The listing builds one solid part. Answer for the finished solid, in the listing's coordinates (mm). Face numbers are marked on the shaded views. A direction names the side the tool comes from. Coordinates: 2 decimals unless noted, no trailing zeros. Write each loop counter-clockwise with the first axis right and the second up, starting at its lowest first coordinate (ties: lowest second). Pieces come first, ordered by that corner, then holes. Notation, with made-up numbers: M 11,43 L 43,43 A37 cw 43,79 Z; hole C 70,77 d10. An arc over 180 degrees is marked long. Answer as CSV lines item,"result".
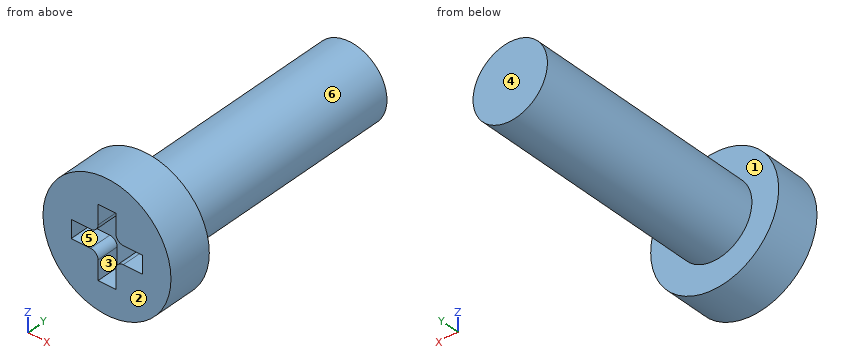
```python
from build123d import *

# Parameters (mm, degrees)
SKETCH_1_R          = 4.3
EXTRUDE_1_DEPTH     = 3
SKETCH_2_R          = 2.5
EXTRUDE_2_DEPTH     = 16
CUT_EXTRUDE_1_DEPTH = 1.5


with BuildPart() as part:
    # 草图1 → 凸台-拉伸1 (new body)
    with BuildSketch(Plane(origin=(0, 0, 0), x_dir=(1, 0, 0), z_dir=(0, 1, 0))):
        Circle(SKETCH_1_R)
    extrude(amount=EXTRUDE_1_DEPTH)

    # 草图2 → 凸台-拉伸2 (add)
    with BuildSketch(Plane(origin=(0, 3, 0), x_dir=(1, 0, 0), z_dir=(0, 1, 0))):
        Circle(SKETCH_2_R)
    extrude(amount=EXTRUDE_2_DEPTH)

    # 草图3 → 切除-拉伸1 (cut)
    with BuildSketch(Plane.XZ):
        with BuildLine():
            Line((-0.6, 1.1), (-0.6, 2.4))
            Line((-0.6, 2.4), (0.6, 2.4))
            Line((0.6, 2.4), (0.6, 1.1))
            ThreePointArc((0.6, 1.1), (0.746446609, 0.746446609), (1.1, 0.6))
            Line((1.1, 0.6), (2.4, 0.6))
            Line((2.4, 0.6), (2.4, -0.6))
            Line((2.4, -0.6), (1.1, -0.6))
            ThreePointArc((1.1, -0.6), (0.746446609, -0.746446609), (0.6, -1.1))
            Line((0.6, -1.1), (0.6, -2.4))
            Line((0.6, -2.4), (-0.6, -2.4))
            Line((-0.6, -2.4), (-0.6, -1.1))
            ThreePointArc((-0.6, -1.1), (-0.746446609, -0.746446609), (-1.1, -0.6))
            Line((-1.1, -0.6), (-2.4, -0.6))
            Line((-2.4, -0.6), (-2.4, 0.6))
            Line((-2.4, 0.6), (-1.1, 0.6))
            ThreePointArc((-1.1, 0.6), (-0.746446609, 0.746446609), (-0.6, 1.1))
        make_face()
    extrude(amount=-CUT_EXTRUDE_1_DEPTH, mode=Mode.SUBTRACT)


solid = part.part
```
Q1. Flat-ended cylindrical pins translate along their axes: pin 1 Ø5 at (x, y) = (1, 10.5) entering from -Z; pin 2 Ø1.5 at (x, y) = (-1, 7.5) entering from +Z; pin 3 Ø4 at (y, z) = (14, 3) entering from +X. Find the tip coordinate at first contact, or state that the pin passes through.
Output:
pin 1,"z = -2.5"
pin 2,"z = 2.49"
pin 3,"x = 2.29"
Q2. The mould has two halves that part along Z. Classify the marked faces 3, 4, 5 and 6: pulls with the +Z half, pulls with the -Z half, needs draft (parallel to the pull), parting line crosses it, or undercut.
Output:
face 3,"undercut"
face 4,"needs draft"
face 5,"undercut"
face 6,"parting line crosses it"
Q3. Find section D-D (z = 3.25). Give the vertices of the cut face in (x, y), and give its area (3 significant figures).
Output:
outline,"M -2.82,0 L 2.82,0 L 2.82,3 L -2.82,3 Z"
area,"16.9 mm2"
Q4. Straight lines are drawn through the part: line 1 (Y direction, x = -3, z = 3); line 2 (Y direction, x = -0.5, z = 0); line 3 (Z direction, x = 0, y = 8). For each, find the intervals that lie inside material, in ascending order.
Output:
line 1,"0 to 3"
line 2,"1.5 to 19"
line 3,"-2.5 to 2.5"
Q5. Find section C-C (y = 14.75). Give the vertices of the cut face in (x, z), and give its area (3 significant figures).
Output:
outline,"C 0,0 d5"
area,"19.6 mm2"
Q6. Find section B-B (z = 0). Give the vertices of the cut face in (x, y).
Output:
outline,"M -4.3,0 L -2.4,0 L -2.4,1.5 L 2.4,1.5 L 2.4,0 L 4.3,0 L 4.3,3 L 2.5,3 L 2.5,19 L -2.5,19 L -2.5,3 L -4.3,3 Z"
Q7. For the marked faces 1 and 2, determine the directions among +Z, -Z, +X, -X, +Y, -Y from which every point of the face is accessible in a straight line to the end or side of a thin tool.
Output:
face 1,"+Y"
face 2,"+Z, -Z, +X, -X, -Y"
Q8. Find section A-A (x = 0). Give the vertices of the cut face in (y, z).
Output:
outline,"M 0,-4.3 L 3,-4.3 L 3,-2.5 L 19,-2.5 L 19,2.5 L 3,2.5 L 3,4.3 L 0,4.3 L 0,2.4 L 1.5,2.4 L 1.5,-2.4 L 0,-2.4 Z"
